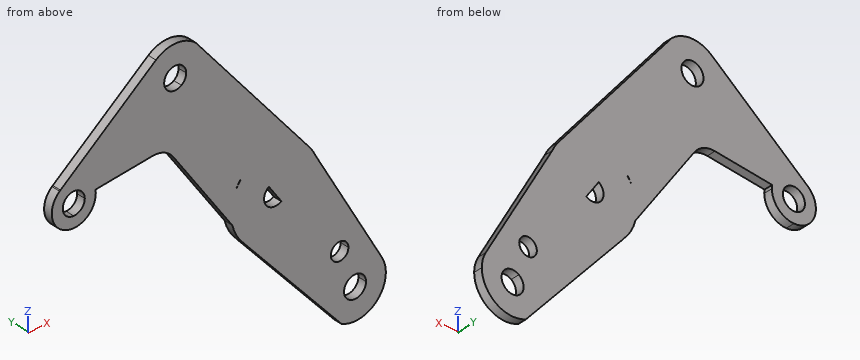
from build123d import *

# Parameters (mm, degrees)
F1_DEPTH = 3.175


# Not quite as in the source:
# - a feature names something its author has since deleted; it is built from what else it names


with BuildPart() as f1:
    # F0 (on Front) → F1 (new body)
    with BuildSketch(Plane.XZ):
        with BuildLine():
            ThreePointArc((41.2067680932, -37.761442646), (34.0261463641, -32.3730062039), (25.2065586875, -34.049743787))
            ThreePointArc((25.2065586875, -34.049743787), (20.9962687571, -39.6141258639), (20.9333080978, -46.5915842229))
            Line((20.9333080978, -46.5915842229), (26.6775649821, -53.2024105477))
            ThreePointArc((26.6775649821, -53.2024105477), (37.4197145601, -52.6119623059), (42.6274718911, -43.1980539644))
            ThreePointArc((42.6274718911, -43.1980539644), (42.2664308978, -40.3884658314), (41.2067680932, -37.761442646))
        make_face()
        with BuildLine():
            ThreePointArc((35.4900718911, -43.1980539644), (29.6668415528, -46.7174053624), (29.258362368, -39.9255727238))
            ThreePointArc((29.258362368, -39.9255727238), (33.3631022294, -39.6787025664), (35.4900718911, -43.1980539644))
        make_face(mode=Mode.SUBTRACT)
        with BuildLine():
            ThreePointArc((20.9333080978, -46.5915842229), (20.9962687571, -39.6141258639), (25.2065586875, -34.049743787))
            Line((25.2065586875, -34.049743787), (23.332877686, -31.3325763437))
            Line((23.332877686, -31.3325763437), (11.7179656145, -14.4889082319))
            Line((11.7179656145, -14.4889082319), (0.788153606, -23.4073638243))
            Line((0.788153606, -23.4073638243), (20.9333080978, -46.5915842229))
        make_face()
        with BuildLine():
            Line((23.332877686, -31.3325763437), (25.2065586875, -34.049743787))
            ThreePointArc((25.2065586875, -34.049743787), (34.0261463641, -32.3730062039), (41.2067680932, -37.761442646))
            Line((41.2067680932, -37.761442646), (17.1943117559, 5.0453389137))
            ThreePointArc((17.1943117559, 5.0453389137), (18.2085059877, 1.9049828695), (18.5515115318, -1.377207439))
            ThreePointArc((18.5515115318, -1.377207439), (17.0177668978, -8.1848516369), (12.7128948986, -13.6770706055))
            Line((12.7128948986, -13.6770706055), (11.7179656145, -14.4889082319))
            Line((11.7179656145, -14.4889082319), (23.332877686, -31.3325763437))
        make_face()
        with BuildLine():
            ThreePointArc((29.1216807586, -29.5301728102), (26.8905558151, -32.5616287109), (23.332877686, -31.3325763437))
            ThreePointArc((23.332877686, -31.3325763437), (25.0028057021, -26.4987169095), (29.1216807586, -29.5301728102))
        make_face(mode=Mode.SUBTRACT)
        with BuildLine():
            Line((0.788153606, -23.4073638243), (11.7179656145, -14.4889082319))
            Line((11.7179656145, -14.4889082319), (11.6885303941, -14.4462219782))
            ThreePointArc((11.6885303941, -14.4462219782), (1.1239010077, -17.1761006141), (-8.7072046251, -12.4418643003))
            Line((-8.7072046251, -12.4418643003), (-8.7249576565, -12.4591197552))
            Line((-8.7249576565, -12.4591197552), (0.788153606, -23.4073638243))
        make_face()
        with BuildLine():
            Line((11.6885303941, -14.4462219782), (11.7179656145, -14.4889082319))
            Line((11.7179656145, -14.4889082319), (12.7128948986, -13.6770706055))
            ThreePointArc((12.7128948986, -13.6770706055), (12.2084738339, -14.0719827293), (11.6885303941, -14.4462219782))
        make_face()
        with BuildLine():
            ThreePointArc((18.5515115318, -1.377207439), (18.2085059877, 1.9049828695), (17.1943117559, 5.0453389137))
            ThreePointArc((17.1943117559, 5.0453389137), (16.2212708068, 6.9025945623), (15.0119525687, 8.6154158115))
            ThreePointArc((15.0119525687, 8.6154158115), (4.9408722756, 14.3354720086), (-6.3355073305, 11.6918071002))
            Line((-6.3355073305, 11.6918071002), (0.4199020087, 1.8952738016))
            ThreePointArc((0.4199020087, 1.8952738016), (4.5246418701, 2.142143959), (6.6516115318, -1.377207439))
            ThreePointArc((6.6516115318, -1.377207439), (6.1958629298, -3.2253377773), (4.9331210549, -4.6496886796))
            Line((4.9331210549, -4.6496886796), (11.6885303941, -14.4462219782))
            ThreePointArc((11.6885303941, -14.4462219782), (12.2084738339, -14.0719827293), (12.7128948986, -13.6770706055))
            ThreePointArc((12.7128948986, -13.6770706055), (17.0177668978, -8.1848516369), (18.5515115318, -1.377207439))
        make_face()
        with BuildLine():
            ThreePointArc((-8.7072046251, -12.4418643003), (1.1239010077, -17.1761006141), (11.6885303941, -14.4462219782))
            Line((11.6885303941, -14.4462219782), (4.9331210549, -4.6496886796))
            ThreePointArc((4.9331210549, -4.6496886796), (2.2877378565, -5.33325029), (-0.1739709939, -4.147797517))
            Line((-0.1739709939, -4.147797517), (-8.7072046251, -12.4418643003))
        make_face()
        with BuildLine():
            ThreePointArc((-6.3355073305, 11.6918071002), (4.9408722756, 14.3354720086), (15.0119525687, 8.6154158115))
            Line((15.0119525687, 8.6154158115), (-23.7631885124, 56.4815721265))
            ThreePointArc((-23.7631885124, 56.4815721265), (-22.6416820928, 53.7897488967), (-22.2590639174, 50.8988507178))
            ThreePointArc((-22.2590639174, 50.8988507178), (-23.5331215108, 45.7323521683), (-27.0631507138, 41.7505405404))
            Line((-27.0631507138, 41.7505405404), (-6.3355073305, 11.6918071002))
        make_face()
        with BuildLine():
            Line((2.6765115318, -1.377207439), (4.9331210549, -4.6496886796))
            ThreePointArc((4.9331210549, -4.6496886796), (6.1958629298, -3.2253377773), (6.6516115318, -1.377207439))
            ThreePointArc((6.6516115318, -1.377207439), (4.5246418701, 2.142143959), (0.4199020087, 1.8952738016))
            Line((0.4199020087, 1.8952738016), (2.6765115318, -1.377207439))
        make_face()
        with BuildLine():
            ThreePointArc((-12.7591425966, -5.0861434898), (-11.2283909413, -9.0367969981), (-8.7072046251, -12.4418643003))
            Line((-8.7072046251, -12.4418643003), (-0.1739709939, -4.147797517))
            ThreePointArc((-0.1739709939, -4.147797517), (-1.2795313193, -0.9884337637), (0.4199020087, 1.8952738016))
            Line((0.4199020087, 1.8952738016), (-6.3355073305, 11.6918071002))
            ThreePointArc((-6.3355073305, 11.6918071002), (-8.12621733, 10.2553621026), (-9.6910264168, 8.5756630059))
            Line((-9.6910264168, 8.5756630059), (-11.3706653491, 6.0182267388))
            ThreePointArc((-11.3706653491, 6.0182267388), (-13.0758245053, 0.5924459256), (-12.7591425966, -5.0861434898))
        make_face()
        with BuildLine():
            ThreePointArc((-9.6910264168, 8.5756630059), (-8.12621733, 10.2553621026), (-6.3355073305, 11.6918071002))
            Line((-6.3355073305, 11.6918071002), (-27.0631507138, 41.7505405404))
            ThreePointArc((-27.0631507138, 41.7505405404), (-35.3796743255, 39.9692968001), (-42.5198740948, 44.5904375142))
            Line((-42.5198740948, 44.5904375142), (-63.4302973575, 30.1712073345))
            ThreePointArc((-63.4302973575, 30.1712073345), (-62.5957178566, 28.6148532084), (-62.125916075, 26.9124879729))
            Line((-62.125916075, 26.9124879729), (-41.4863105467, 29.2003405071))
            ThreePointArc((-41.4863105467, 29.2003405071), (-37.3081114888, 28.5304448001), (-34.0654515171, 25.8117568934))
            Line((-34.0654515171, 25.8117568934), (-15.783328424, -0.7005414231))
            Line((-15.783328424, -0.7005414231), (-11.3706653491, 6.0182267388))
            ThreePointArc((-11.3706653491, 6.0182267388), (-10.5926033575, 7.337505124), (-9.6910264168, 8.5756630059))
        make_face()
        with BuildLine():
            ThreePointArc((-22.2590639174, 50.8988507178), (-22.6416820928, 53.7897488967), (-23.7631885124, 56.4815721265))
            Line((-23.7631885124, 56.4815721265), (-25.9160326978, 59.1391608141))
            ThreePointArc((-25.9160326978, 59.1391608141), (-33.0370839347, 62.0063157477), (-40.3177534576, 59.572840983))
            ThreePointArc((-40.3177534576, 59.572840983), (-44.3659412857, 52.514809422), (-42.5198740948, 44.5904375142))
            Line((-42.5198740948, 44.5904375142), (-36.644045158, 48.6422411947))
            ThreePointArc((-36.644045158, 48.6422411947), (-34.5532956616, 54.6942334514), (-29.3964639174, 50.8988507178))
            ThreePointArc((-29.3964639174, 50.8988507178), (-29.8522125194, 49.0507203795), (-31.1149543943, 47.6263694772))
            Line((-31.1149543943, 47.6263694772), (-27.0631507138, 41.7505405404))
            ThreePointArc((-27.0631507138, 41.7505405404), (-23.5331215108, 45.7323521683), (-22.2590639174, 50.8988507178))
        make_face()
        with BuildLine():
            Line((-15.783328424, -0.7005414231), (-12.7591425966, -5.0861434898))
            ThreePointArc((-12.7591425966, -5.0861434898), (-13.0758245053, 0.5924459256), (-11.3706653491, 6.0182267388))
            Line((-11.3706653491, 6.0182267388), (-15.783328424, -0.7005414231))
        make_face()
        with BuildLine():
            ThreePointArc((-42.5198740948, 44.5904375142), (-35.3796743255, 39.9692968001), (-27.0631507138, 41.7505405404))
            Line((-27.0631507138, 41.7505405404), (-31.1149543943, 47.6263694772))
            ThreePointArc((-31.1149543943, 47.6263694772), (-34.0898936977, 46.989193145), (-36.644045158, 48.6422411947))
            Line((-36.644045158, 48.6422411947), (-42.5198740948, 44.5904375142))
        make_face()
        with BuildLine():
            Line((-63.4302973575, 30.1712073345), (-42.5198740948, 44.5904375142))
            ThreePointArc((-42.5198740948, 44.5904375142), (-44.3659412857, 52.514809422), (-40.3177534576, 59.572840983))
            Line((-40.3177534576, 59.572840983), (-74.7776425006, 31.9771308762))
            ThreePointArc((-74.7776425006, 31.9771308762), (-68.717256497, 33.5040453897), (-63.4302973575, 30.1712073345))
        make_face()
        with BuildLine():
            ThreePointArc((-62.125916075, 26.9124879729), (-62.5957178566, 28.6148532084), (-63.4302973575, 30.1712073345))
            Line((-63.4302973575, 30.1712073345), (-66.6923233865, 27.9218074265))
            ThreePointArc((-66.6923233865, 27.9218074265), (-66.1694218935, 26.8469296476), (-65.9897046271, 25.6651979034))
            ThreePointArc((-65.9897046271, 25.6651979034), (-67.1539844612, 22.8543777375), (-69.9648046271, 21.6900979034))
            Line((-69.9648046271, 21.6900979034), (-69.9648046271, 17.7276979034))
            ThreePointArc((-69.9648046271, 17.7276979034), (-64.3521445515, 20.0525378277), (-62.0273046271, 25.6651979034))
            ThreePointArc((-62.0273046271, 25.6651979034), (-62.0519958928, 26.2907889709), (-62.125916075, 26.9124879729))
        make_face()
        with BuildLine():
            Line((-66.6923233865, 27.9218074265), (-63.4302973575, 30.1712073345))
            ThreePointArc((-63.4302973575, 30.1712073345), (-68.717256497, 33.5040453897), (-74.7776425006, 31.9771308762))
            Line((-74.7776425006, 31.9771308762), (-75.0722889717, 31.7411760073))
            ThreePointArc((-75.0722889717, 31.7411760073), (-77.4224175981, 22.9471259719), (-69.9648046271, 17.7276979034))
            Line((-69.9648046271, 17.7276979034), (-69.9648046271, 21.6900979034))
            ThreePointArc((-69.9648046271, 21.6900979034), (-73.4841560252, 27.5133282417), (-66.6923233865, 27.9218074265))
        make_face()
    extrude(amount=F1_DEPTH)


solid = f1.part
Part model, mm, in its own coordinate system. Round coordinates to 2 decimals unless told otherwise and drop trailing zeros. Write each loop counter-clockwise with the first axis right and the second up, starting at its lowest first coordinate (ties: lowest second). Pieces come first, ordered by that corner, then holes. Notation, with made-up numbers: M 26,41 L 43,41 A28 ccw 43,77 Z; hole C -35,-4 d10. An arc over 180 degrees is marked long. Return JSON: item names as keys, results as strings. Group by question number.
(1) Drill centre lines: probe 1 along X at (y, z) = (-2.9, 23.5); probe 2 along X at (y, z) = (-2.85, 18.5); probe 3 along Z at (x, y) = (35, -1.15). Where is each one in solid material? Low to high.
(2) Pin check, flat tip, straight feed: pin 1 Ø1.5 at (x, y) = (2.5, -2.5) entering from +Z. Stop position of the tip, or through.
(3) Saw through at B-B on x = 32.5. Write the cut outline in (y, z) (3 decimals), then the cut area to 3 significant figures.
(4) Saw through at C-C on z = 40. Write the cut outline in (x, y) (3 decimals).
(5) Saw through at A-A on y = -1.85. Count the separate pieces of the cut face and the enclosed holes in it, then the cut area to 3 significant figures.
(6) Saw through at D-D on x = -54. Write the cut outline in (y, z) (3 decimals).
Returned:
{
 "1": {"probe 1": "-77.6 to -73.3, -66.63 to -62.33, -32.47 to 2.95", "probe 2": "-73.38 to -66.55, -29.02 to 7", "probe 3": "-53.75 to -45.11, -41.29 to -26.7"},
 "2": {"pin 1": "z = 24.99"},
 "3": {"outline": "M -3.175,-54.267 L 0,-54.267 L 0,-47.049 L -3.175,-47.049 Z; M -3.175,-39.347 L 0,-39.347 L 0,-22.24 L -3.175,-22.24 Z", "area": "77.2 mm²"},
 "4": {"outline": "M -64.759,-3.175 L -10.412,-3.175 L -10.412,0 L -64.759,0 Z"},
 "5": {"separate pieces": "1", "enclosed holes": "6", "area": "4,020 mm²"},
 "6": {"outline": "M -3.175,27.813 L 0,27.813 L 0,48.616 L -3.175,48.616 Z"}
}
